Geometry check sheet. Reference: the model listing, model coordinates, mm. Face numbers are marked on the shaded views. A direction names the side the tool comes from. Coordinates: 2 decimals unless noted, no trailing zeros. Loops run counter-clockwise (first coordinate to the right, second up) from the corner with the lowest first, then second, coordinate; pieces in that order, holes last. Notation, with made-up numbers: M 27.5,17 L 38.5,17 A14 cw 38.5,31 Z; hole C 60,45 d8. An arc over 180 degrees is marked long. One line per question, with ' | ' between items. Start each with the question number.
from build123d import *

# Parameters (mm, degrees)
SKETCH1_W               = 33.3
SKETCH1_H               = 48.3
BOSS_EXTRUDE1_DEPTH     = 9.55
CUT_EXTRUDE1_DEPTH      = 5
CUT_EXTRUDE2_DEPTH      = 4.5
SKETCH5_W               = 33.3
SKETCH5_H               = 48.3
BOSS_EXTRUDE3_DEPTH     = 22.5
SKETCH6_R               = 4.025
CUT_EXTRUDE3_DEPTH      = 12
SKETCH7_R               = 4.125
CUT_EXTRUDE4_DEPTH      = 15.05
CUT_EXTRUDE6_DEPTH      = 46.909857329
CUT_EXTRUDE6_DEPTH_BACK = 46.909857329
SKETCH27_R              = 1.5
SKETCH30_R              = 4
SKETCH31_R              = 5
CHAMFER1_SIZE           = 13
CHAMFER1_SIZE2          = 7.505553499
CHAMFER2_SIZE           = 10
CHAMFER2_SIZE2          = 17.320508076
CHAMFER3_SIZE           = 3
CHAMFER3_SIZE2          = 1.732050808


with BuildPart() as part:
    # Sketch1 → Boss-Extrude1 (new body)
    with BuildSketch(Plane(origin=(0, 0, 0), x_dir=(0, 0, -1), z_dir=(1, 0, 0))):
        Rectangle(SKETCH1_W, SKETCH1_H)
    extrude(amount=BOSS_EXTRUDE1_DEPTH)

    # Sketch2 → Cut-Extrude1 (cut)
    with BuildSketch(Plane.ZY):
        Polygon((0, 19.15), (-5.65, 19.15), (-5.65, 5.45), (-11.65, -0.987390776), (-11.65, -9.1), (-10.577101537, -10.1), (10.577101537, -10.1), (11.65, -9.1), (11.65, -0.987390776), (5.65, 5.45), (5.65, 11.45), (4.5, 12.6), (4.5, 19.15), align=None)
    extrude(amount=-CUT_EXTRUDE1_DEPTH, mode=Mode.SUBTRACT)

    # Sketch3 → Cut-Extrude2 (cut)
    with BuildSketch(Plane.ZY.offset(-5)):
        Polygon((-5.65, 19.15), (4.5, 19.15), (4.5, 12.6), (5.65, 11.45), (5.65, 5.45), (-5.65, 5.45), align=None)
    extrude(amount=-CUT_EXTRUDE2_DEPTH, mode=Mode.SUBTRACT)

    # Sketch5 → Boss-Extrude3 (add)
    with BuildSketch(Plane(origin=(9.55, 0, 0), x_dir=(0, 0, -1), z_dir=(1, 0, 0))):
        Rectangle(SKETCH5_W, SKETCH5_H)
    extrude(amount=BOSS_EXTRUDE3_DEPTH)

    # Sketch6 → Cut-Extrude3 (cut)
    with BuildSketch(Plane.ZY.offset(-5)):
        with Locations((0, -2.575)):
            Circle(SKETCH6_R)
    extrude(amount=-CUT_EXTRUDE3_DEPTH, mode=Mode.SUBTRACT)

    # Sketch7 → Cut-Extrude4 (cut)
    with BuildSketch(Plane.ZY.offset(-17)):
        with Locations((0, -2.575)):
            Circle(SKETCH7_R)
    extrude(amount=-CUT_EXTRUDE4_DEPTH, mode=Mode.SUBTRACT)

    # Sketch27 → Cut-Extrude6 (cut, two sides: drawn at the far end of the back side and taken through both)
    with BuildSketch(Plane(origin=(0, 0, 5.65), x_dir=(-1, 0, 0), z_dir=(0, 0, -1)).offset(-CUT_EXTRUDE6_DEPTH_BACK)):
        with Locations((-7, 7.95)):
            Circle(SKETCH27_R)
    extrude(amount=CUT_EXTRUDE6_DEPTH + CUT_EXTRUDE6_DEPTH_BACK, mode=Mode.SUBTRACT)

    # Cut-Sweep1: sweep along a path in Sketch28
    with BuildLine(Plane.XY) as cut_sweep1_path:
        Line((25.361872918, -28.011391971), (13, -6.6))
        Line((13, -6.6), (10.184139233, -1.722786085))
    # Sketch30 → Cut-Sweep1 (sweep, cut)
    with BuildSketch(Plane(origin=(18.469756751, -31.990557096, 0), x_dir=(0, 0, -1), z_dir=(0.500000000000001, -0.866025403784438, 0))):
        with Locations((0, 7.958330249)):
            Circle(SKETCH30_R)
    sweep(path=cut_sweep1_path.line, mode=Mode.SUBTRACT)

    # Cut-Sweep2: sweep along a path in Sketch29
    with BuildLine(Plane.XY) as cut_sweep2_path:
        Line((19, -16.992304845), (25.361872918, -28.011391971))
    # Sketch31 → Cut-Sweep2 (sweep, cut)
    with BuildSketch(Plane(origin=(18.469756751, -31.990557096, 0), x_dir=(0, 0, -1), z_dir=(0.500000000000001, -0.866025403784438, 0))):
        with Locations((0, 7.958330249)):
            Circle(SKETCH31_R)
    sweep(path=cut_sweep2_path.line, mode=Mode.SUBTRACT)

    # Chamfer1
    chamfer1_edges = [part.edges().sort_by_distance(p)[0] for p in [
        (0, -24.15, 0),
    ]]
    chamfer1_side = [part.faces().sort_by_distance(p)[0] for p in [
        (0, 23.563333144, 0),
    ]]
    chamfer(chamfer1_edges, length=CHAMFER1_SIZE, length2=CHAMFER1_SIZE2, reference=chamfer1_side[0])

    # Chamfer2
    chamfer2_edges = [part.edges().sort_by_distance(p)[0] for p in [
        (32.05, 24.15, 0),
    ]]
    chamfer2_side = [part.faces().sort_by_distance(p)[0] for p in [
        (16.025, 24.15, 0),
    ]]
    chamfer(chamfer2_edges, length=CHAMFER2_SIZE, length2=CHAMFER2_SIZE2, reference=chamfer2_side[0])

    # Chamfer3
    chamfer3_edges = [part.edges().sort_by_distance(p)[0] for p in [
        (32.05, -24.15, 0),
    ]]
    chamfer3_side = [part.faces().sort_by_distance(p)[0] for p in [
        (19.77777675, -24.15, -16.236318981),
    ]]
    chamfer(chamfer3_edges, length=CHAMFER3_SIZE, length2=CHAMFER3_SIZE2, reference=chamfer3_side[0])


solid = part.part
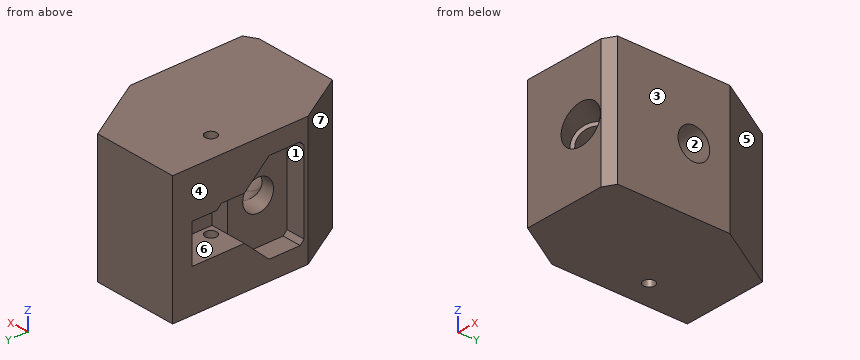
1. Sectioned sample at B-B (z = 0). Record the cut outline in (x, y), and give its area (3 significant figures).
2. Thickness scan on line 1 (Z direction, x = 5, y = 6.5); line 2 (Z direction, x = 2.5, y = 14.5); line 3 (X direction, y = -2.5, z = 8). Record the ranges inside material, lowest first.
3. Draft check along Y on the marked faces 4, 5, 6 and 7. Enter one of: +Y half, -Y half, draft (parallel to the pull), parting line (faces both ways), or undercut.
4. Sectioned sample at C-C (y = 15.5). Record the cut outline in (x, z).
5. Tool access check on the marked faces 1, 2 and 3. Record the directions out of +Z, -Z, +X, -X, +Y, -Y that give a thin tool (end or side, any length) a straight path to the whole face; none if there is none.
6. Sectioned sample at D-D (x = 4). Record the cut outline in (y, z).
7. Sectioned sample at A-A (z = 14.5). Record the cut outline in (x, y).
8. Depth check by flat-ended pin: pin 1 Ø17 at (y, z) = (-0.5, -3.5) entering from -X; pin 2 Ø4 at (y, z) = (17, -3) entering from +X; pin 3 Ø2.5 at (x, y) = (7, 7.95) entering from +Z. Enter the tip coordinate at first touch or a pass-through.
Result:
1) outline: M 0,-11.15 L 7.51,-24.15 L 17.36,-24.15 L 14.67,-19.49 L 15.54,-18.99 L 8.38,-6.6 L 5,-6.6 L 5,-10.1 L 0,-10.1 Z; M 0,19.15 L 9.5,19.15 L 9.5,5.45 L 5,5.45 L 5,1.45 L 17,1.45 L 17,1.55 L 32.05,1.55 L 32.05,6.83 L 22.05,24.15 L 0,24.15 Z; M 17.68,-6.7 L 22.46,-14.99 L 23.33,-14.49 L 28.91,-24.15 L 29.05,-24.15 L 32.05,-22.42 L 32.05,-6.7 Z | area: 803 mm2
2) line 1: z = -16.65 to -5.65, 5.65 to 16.65 | line 2: z = -16.65 to -5.65, 4.5 to 16.65 | line 3: x = 5 to 32.05
3) face 4: draft | face 5: +Y half | face 6: undercut | face 7: -Y half
4) outline: M 0,-16.65 L 27.04,-16.65 L 27.04,16.65 L 0,16.65 L 0,4.5 L 9.5,4.5 L 9.5,-5.65 L 0,-5.65 Z
5) face 1: -X | face 2: +X | face 3: +Z, -Z, +X, +Y, -Y
6) outline: M -18.08,-16.65 L 24.15,-16.65 L 24.15,16.65 L -18.08,16.65 Z; hole M -10.1,-10.58 L -9.1,-11.65 L -0.99,-11.65 L 5.45,-5.65 L 19.15,-5.65 L 19.15,4.5 L 12.6,4.5 L 11.45,5.65 L 5.45,5.65 L -0.99,11.65 L -9.1,11.65 L -10.1,10.58 Z
7) outline: M 0,-11.15 L 7.51,-24.15 L 29.05,-24.15 L 32.05,-22.42 L 32.05,6.83 L 22.05,24.15 L 0,24.15 Z; hole C 7,7.95 d3
8) pin 1: stops at x = 0 | pin 2: stops at x = 27.33 | pin 3: passes through
